Check sheet for the modelled part. Datum: model origin and axes. Units: mm. A direction names the side the tool comes from. Give positions to 0.01 mm unless a question says otherwise; leave off trailing zeros. Write each loop counter-clockwise with the first axis right and the second up, starting at its lowest first coordinate (ties: lowest second). Pieces come first, ordered by that corner, then holes. Notation, with made-up numbers: (34, -27) -> (78, -27) arc R20 ccw to (78, 11) -> close; hole circle Ø3 at (14.5, 16). An arc over 180 degrees is marked (long way). Return JSON: item names as keys, results as strings.
from build123d import *

# Parameters (mm, degrees)
SKETCH1_W                = 48
SKETCH1_H                = 71
SKETCH1_W_2              = 42
SKETCH1_H_2              = 65
BOSS_EXTRUDE1_DEPTH      = 80
M3_CLEARANCE_HOLE1_D     = 3.4
M3_CLEARANCE_HOLE1_DEPTH = 3
SKETCH5_W                = 8
SKETCH5_H                = 3
CUT_EXTRUDE1_DEPTH       = 110.622078068
FILLET1_R                = 2
FILLET2_R                = 1


with BuildPart() as part:
    # Sketch1 → Boss-Extrude1 (new body)
    with BuildSketch(Plane(origin=(0, 0, 0), x_dir=(1, 0, 0), z_dir=(0, 1, 0))):
        Rectangle(SKETCH1_W, SKETCH1_H)
        Rectangle(SKETCH1_W_2, SKETCH1_H_2, mode=Mode.SUBTRACT)
    extrude(amount=BOSS_EXTRUDE1_DEPTH)

    # M3 Clearance Hole1
    with Locations(Plane(origin=(-21, 0, 0), x_dir=(0, 0, -1), z_dir=(1, 0, 0))):
        with Locations((0, 40), (0, 47), (7, 40), (0, 33), (-7, 40)):
            Hole(M3_CLEARANCE_HOLE1_D / 2, depth=M3_CLEARANCE_HOLE1_DEPTH)

    # Sketch5 → Cut-Extrude1 (cut, through all)
    with BuildSketch(Plane.XY.offset(35.5)):
        with Locations((0, 4.5)):
            Rectangle(SKETCH5_W, SKETCH5_H)
        with Locations((0, 75.5)):
            Rectangle(SKETCH5_W, SKETCH5_H)
        with Locations((14, 4.5)):
            Rectangle(SKETCH5_W, SKETCH5_H)
        with Locations((-14, 4.5)):
            Rectangle(SKETCH5_W, SKETCH5_H)
        with Locations((-14, 75.5)):
            Rectangle(SKETCH5_W, SKETCH5_H)
        with Locations((14, 75.5)):
            Rectangle(SKETCH5_W, SKETCH5_H)
    extrude(amount=-CUT_EXTRUDE1_DEPTH, mode=Mode.SUBTRACT)

    # Fillet1
    fillet1_edges = [part.edges().sort_by_distance(p)[0] for p in [
        (21, 40, 32.5),
        (21, 40, -32.5),
        (-21, 40, -32.5),
        (-21, 40, 32.5),
        (-24, 40, -35.5),
        (24, 40, -35.5),
        (24, 40, 35.5),
        (-24, 40, 35.5),
    ]]
    fillet(fillet1_edges, radius=FILLET1_R)

    # Fillet2
    fillet2_edges = [part.edges().sort_by_distance(p)[0] for p in [
        (-4, 74, -34),
        (-4, 77, -34),
        (4, 77, -34),
        (4, 74, -34),
        (-4, 74, 34),
        (-4, 77, 34),
        (4, 77, 34),
        (4, 74, 34),
        (18, 6, -34),
        (18, 3, -34),
        (10, 3, -34),
        (10, 6, -34),
        (18, 6, 34),
        (18, 3, 34),
        (10, 3, 34),
        (10, 6, 34),
        (-10, 6, -34),
        (-10, 3, -34),
        (-18, 3, -34),
        (-18, 6, -34),
        (-10, 6, 34),
        (-10, 3, 34),
        (-18, 3, 34),
        (-18, 6, 34),
        (-18, 74, -34),
        (-18, 77, -34),
        (-10, 77, -34),
        (-10, 74, -34),
        (-18, 74, 34),
        (-18, 77, 34),
        (-10, 77, 34),
        (-10, 74, 34),
        (10, 74, -34),
        (10, 77, -34),
        (18, 77, -34),
        (18, 74, -34),
        (10, 74, 34),
        (10, 77, 34),
        (18, 77, 34),
        (18, 74, 34),
        (4, 6, -34),
        (4, 3, -34),
        (-4, 3, -34),
        (-4, 6, -34),
        (4, 6, 34),
        (4, 3, 34),
        (-4, 3, 34),
        (-4, 6, 34),
    ]]
    fillet(fillet2_edges, radius=FILLET2_R)


solid = part.part
(1) Set-up check for faces 4 (the cylindrical face through (-20.4, 40.56, -31.93)), 5 (the flat face through (-21.4, 80, -2.8)), 6 (the flat face through (0, 3, -34)): record each of +Z, -Z, +X, -X, +Y, -Y from which the full face is reachable in a straight line by a thin tool's end or side.
Reply:
{"face 4": "+Y, -Y", "face 5": "+Z, -Z, +X, -X, +Y", "face 6": "+Z, -Z"}
(2) Thickness scan on L1, parallel to Y at x = -23, z = 0; L2, parallel to Z at x = -9, y = 35; L3, parallel to X at y = 4.5, z = 21.5. Record the ranges inside material, lowest first.
Reply:
{"L1": "0 to 31.3, 34.7 to 38.3, 41.7 to 45.3, 48.7 to 80", "L2": "-35.5 to -32.5, 32.5 to 35.5", "L3": "-24 to -21, 21 to 24"}
(3) Cross-section at B-B on y = 24.5. Enter the section's corners in (x, z), then the cut area to 3 significant figures.
Reply:
{"outline": "(-24, -33.5) arc R2 ccw to (-22, -35.5) -> (22, -35.5) arc R2 ccw to (24, -33.5) -> (24, 33.5) arc R2 ccw to (22, 35.5) -> (-22, 35.5) arc R2 ccw to (-24, 33.5) -> close; hole (-21, -30.5) arc R2 ccw to (-19, -32.5) -> (19, -32.5) arc R2 ccw to (21, -30.5) -> (21, 30.5) arc R2 ccw to (19, 32.5) -> (-19, 32.5) arc R2 ccw to (-21, 30.5) -> close", "area": "678 mm^2"}
(4) Release check for a two-part mould opening along X. For faces 1 (the cylindrical face through (20.43, 40.56, -31.9)), 2 (the cylindrical face through (23.4, 40.56, 34.93)), 3 (the cylindrical face through (-22.52, 31.34, -0.37)) record: pulls with the +X half, pulls with the -X half, needs draft (parallel to the pull), parting line crosses it, or undercut.
Reply:
{"face 1": "undercut", "face 2": "pulls with the +X half", "face 3": "needs draft"}
(5) Cross-section at A-A on z = 0. Enter the section's corners in (x, y), then the cut area to 3 significant figures.
Reply:
{"outline": "(-24, 0) -> (-21, 0) -> (-21, 31.3) -> (-24, 31.3) -> close; (-24, 34.7) -> (-21, 34.7) -> (-21, 38.3) -> (-24, 38.3) -> close; (-24, 41.7) -> (-21, 41.7) -> (-21, 45.3) -> (-24, 45.3) -> close; (-24, 48.7) -> (-21, 48.7) -> (-21, 80) -> (-24, 80) -> close; (21, 0) -> (24, 0) -> (24, 80) -> (21, 80) -> close", "area": "449 mm^2"}
(6) Cross-section at C-C on x = -16. Enter the section's corners in (y, z).
Reply:
{"outline": "(0, -35.5) -> (3, -35.5) -> (3, -32.5) -> (0, -32.5) -> close; (0, 32.5) -> (3, 32.5) -> (3, 35.5) -> (0, 35.5) -> close; (6, -35.5) -> (74, -35.5) -> (74, -32.5) -> (6, -32.5) -> close; (6, 32.5) -> (74, 32.5) -> (74, 35.5) -> (6, 35.5) -> close; (77, -35.5) -> (80, -35.5) -> (80, -32.5) -> (77, -32.5) -> close; (77, 32.5) -> (80, 32.5) -> (80, 35.5) -> (77, 35.5) -> close"}
(7) Cross-section at D-D on z = 20. Enter the section's corners in (x, y).
Reply:
{"outline": "(-24, 0) -> (-21, 0) -> (-21, 80) -> (-24, 80) -> close; (21, 0) -> (24, 0) -> (24, 80) -> (21, 80) -> close"}
(8) Depth check by flat-ended pin: pin 1 Ø0.8 at (y, z) = (4.5, 34.5) entering from +X; pin 2 Ø0.9 at (x, z) = (0.5, -34) entering from -Y; pin 3 Ø0.8 at (y, z) = (75.5, 34) entering from -X; pin 4 Ø2.5 at (y, z) = (40, 0) entering from -X. Enter the tip coordinate at first touch or a pass-through.
Reply:
{"pin 1": "x = 23.91", "pin 2": "y = 0", "pin 3": "x = -24", "pin 4": "x = 21"}
